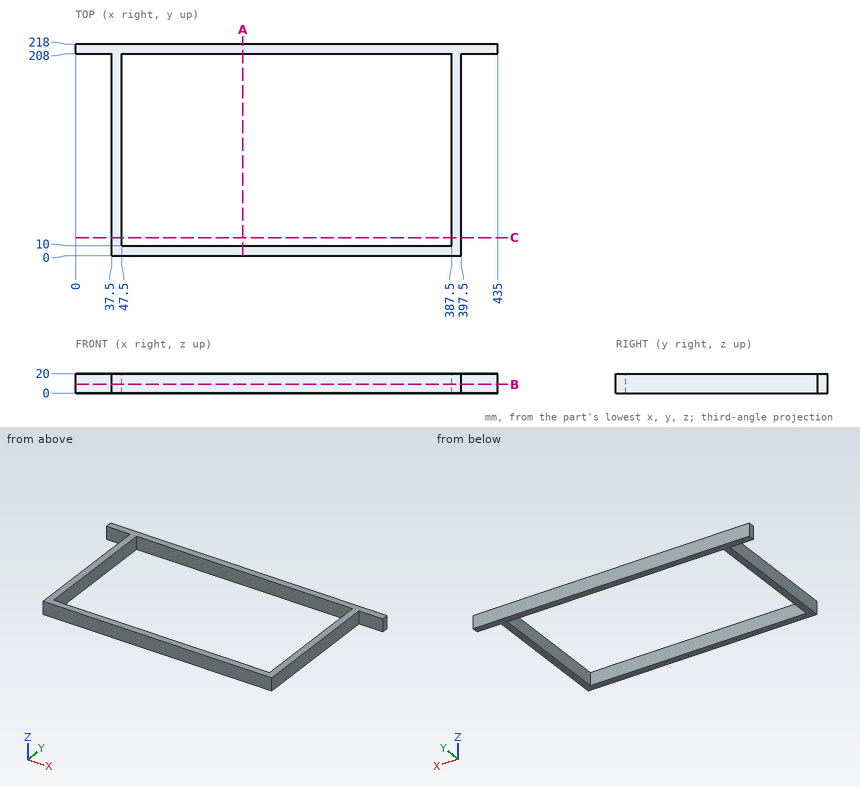
Input: dimensioned drawing with shaded views. Units: mm. Origin: part minimum x, y, z. Round coordinates to 2 decimals unless told otherwise and drop trailing zeros. Order: outer loops, then holes, each group sorted by start corner. A loop starts at its lowest first (then second) coordinate and runs counter-clockwise, first axis right, second up. Notation, with made-up numbers: (12, 85.5) - (22, 85.5) arc R25 ccw to (22, 100.5) - close; hole circle Ø2 at (-11.75, -36.75). An arc over 180 degrees is marked (long way). Use CSV: the item, a comma, the result in double quotes. Start each with the question number.
Q1. First-contact query: pin 1 (1 mm diameter, centred on y = 99, z = 12.5, fed in from +X); pin 2 (6 mm diameter, centred on x = 18.5, z = 13, fed in from -Y); pin 3 (3 mm diameter, centred on y = 145.5, z = 12, fed in from -X). Flat tips, straight axial feed; report the tip coordinate or a pass-through.
Q2. Section query A-A (x = 172.5). Return loops of the section in (y, z).
Q3. Section query C-C (y = 18.5). Return loops of the section in (x, z).
Q4. Material intervals for line 1 along Y through (x, z) = (243.5, 15); line 2 along X through (y, z) = (72, 7.75); line 3 along Y through (x, z) = (413, 14.5), sorted ascending. Write a range as from..to.
Q5. Section query B-B (z = 9). Return loops of the section in (x, y).
Result set:
1,pin 1,"stops at x = 397.5"
1,pin 2,"stops at y = 208"
1,pin 3,"stops at x = 37.5"
2,outline,"(0, 0) - (10, 0) - (10, 20) - (0, 20) - close; (208, 0) - (218, 0) - (218, 20) - (208, 20) - close"
3,outline,"(37.5, 0) - (47.5, 0) - (47.5, 20) - (37.5, 20) - close; (387.5, 0) - (397.5, 0) - (397.5, 20) - (387.5, 20) - close"
4,line 1,"y = 0..10, 208..218"
4,line 2,"x = 37.5..47.5, 387.5..397.5"
4,line 3,"y = 208..218"
5,outline,"(0, 208) - (37.5, 208) - (37.5, 0) - (397.5, 0) - (397.5, 208) - (435, 208) - (435, 218) - (0, 218) - close; hole (47.5, 10) - (387.5, 10) - (387.5, 208) - (47.5, 208) - close"
